```python
from build123d import *

# Parameters (mm, degrees)
BOX001_W               = 2
BOX001_H               = 10
BOX001_DEPTH           = 2
BOX001_ROLL_ANGLE      = -0.060026
BOX001_PITCH_ANGLE     = 1.435067
BOX001_PLACEMENT_ANGLE = -4.790134
BOX_W                  = 2
BOX_H                  = 10
BOX_DEPTH              = 2
BOX_PLACEMENT_ANGLE    = 45


with BuildPart() as cubo001:
    # Box001 → Box001 (new body)
    with BuildSketch(Plane.XY):
        with Locations((1, 5)):
            Rectangle(BOX001_W, BOX001_H)
    extrude(amount=BOX001_DEPTH)


with BuildPart() as cubo001_1:
    # Box001 roll: moved
    add(cubo001.part.rotate(Axis((0, 0, 0), (1, 0, 0)), BOX001_ROLL_ANGLE))


with BuildPart() as cubo001_2:
    # Box001 pitch: moved
    add(cubo001_1.part.rotate(Axis((0, 0, 0), (0, 1, 0)), BOX001_PITCH_ANGLE))


with BuildPart() as cubo001_3:
    # Box001 placement: moved
    add(cubo001_2.part.moved(Location((3, 2, 0))).rotate(Axis((3, 2, 0), (0, 0, 1)), BOX001_PLACEMENT_ANGLE))


with BuildPart() as fusion:
    # Box → Box (new body)
    with BuildSketch(Plane.XY):
        with Locations((1, 5)):
            Rectangle(BOX_W, BOX_H)
    extrude(amount=BOX_DEPTH)


with BuildPart() as fusion_1:
    # Box placement: moved
    add(fusion.part.moved(Location((7, 3, 0))).rotate(Axis((7, 3, 0), (0, 0, 1)), BOX_PLACEMENT_ANGLE))

    # Fusion: union Cubo001
    add(cubo001_3.part)


solid = fusion_1.part
```
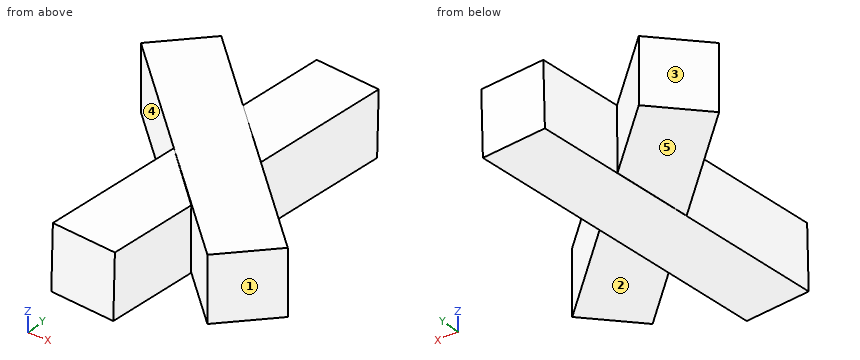
Here's how the part is built. I have some questions about the finished solid (model axes, mm). Face numbers are marked on the shaded views. A direction names the side the tool comes from. Round coordinates to 2 decimals unless told otherwise and drop trailing zeros. Loops run counter-clockwise (first coordinate to the right, second up) from the corner with the lowest first, then second, coordinate; pieces in that order, holes last. Notation, with made-up numbers: (12, 76.5) -> (25, 76.5) arc R24 cw to (25, 92.5) -> close; hole circle Ø10 at (51, 24.25). An arc over 180 degrees is marked (long way). Answer as CSV lines item,"result". Start each with the question number.
1. I'm going to push flat-ended pins straight in: P1, Ø3, axis at x = 3, y = 5, coming from the +Z side; P2, Ø3, axis at x = 2, y = 9, coming from the -Z side; P3, Ø2.5, axis at x = 6.5, y = 5.5, coming from the -Z side. Where does each tip first touch, or does it pass through?
2. Imagine slicing it at B-B on x = 3.25. Write out the boundary of the cut face in (y, z).
3. Imagine slicing it at A-A on y = 9.5. Write out the boundary of the cut face in (x, z).
4. I need wall thicknesses on probe 1 along Z at (x, y) = (3.5, 4); probe 2 along X at (y, z) = (4, 0.9); probe 3 along Y at (x, z) = (4.25, 0.5). Which ranges of each line are inside material? Lowest first, please. Write a range as from..to.
5. Imagine slicing it at C-C on z = 0.4. Write out the boundary of the cut face in (x, y), plus the area to 3 significant figures.
6. For the marked faces 1 and 2, which set-ups out of +Z, -Z, +X, -X, +Y, -Y let a thin tool reach every point of the face, with its end or its side?
7. If we mould it in two halves opening along X, with no side actions, what happens to the marked faces 3, 4 and 5? For each: pulls with the +X half, pulls with the -X half, needs draft (parallel to the pull), parting line crosses it, or undercut.
Solution:
1,P1,"z = 2"
1,P2,"z = 0"
1,P3,"z = -0.05"
2,outline,"(1.98, -0.01) -> (4.98, 0) -> (4.38, 2) -> (1.98, 1.99) -> close; (6.75, 0) -> (9.58, 0) -> (9.58, 2) -> (6.75, 2) -> close"
3,outline,"(0.5, 0) -> (3.33, 0) -> (3.33, 2) -> (0.5, 2) -> close; (3.63, -0.01) -> (5.63, -0.06) -> (5.68, 1.94) -> (3.68, 1.99) -> close"
4,probe 1,"-0.01..1.99"
4,probe 2,"3.19..5.2, 6..8"
4,probe 3,"1.9..11.93"
5,outline,"(-0.07, 10.07) -> (3.4, 6.6) -> (3.01, 2) -> (5, 1.83) -> (5.25, 4.75) -> (7, 3) -> (8.41, 4.41) -> (5.47, 7.36) -> (5.84, 11.8) -> (3.85, 11.96) -> (3.61, 9.21) -> (1.34, 11.49) -> close"
5,area,"34.8 mm²"
6,face 1,"+Z, -Z, +X, -Y"
6,face 2,"-Z, +X, -Y"
7,face 3,"pulls with the -X half"
7,face 4,"undercut"
7,face 5,"needs draft"
